```python
from build123d import *

# Parameters (mm, degrees)
F0_W     = 50.8
F0_H     = 38.1
F1_DEPTH = 50.8
F2_R     = 4.7625
F3_DEPTH = 50.801
F4_R     = 4.7625
F5_DEPTH = 38.101
F6_R     = 2.54
F7_DEPTH = 12.7
F8_R     = 2.54
F9_DEPTH = 19.05


with BuildPart() as f1:
    # F0 (on Front) → F1 (new body)
    with BuildSketch(Plane.XZ):
        Rectangle(F0_W, F0_H)
    extrude(amount=F1_DEPTH)

    # F2 (on face) → F3 (cut, through all)
    with BuildSketch(Plane(origin=(0, 0, 0), x_dir=(-1, 0, 0), z_dir=(0, 1, 0))):
        with Locations((-4.7625, 0)):
            Circle(F2_R)
    extrude(amount=-F3_DEPTH, mode=Mode.SUBTRACT)

    # F4 (on face) → F5 (cut, through all)
    with BuildSketch(Plane.XY.offset(19.05)):
        with Locations((-12.7, -25.4)):
            Circle(F4_R)
    extrude(amount=-F5_DEPTH, mode=Mode.SUBTRACT)

    # F6 (on face) → F7 (cut)
    with BuildSketch(Plane(origin=(-25.4, 0, 0), x_dir=(0, -1, 0), z_dir=(-1, 0, 0))):
        with Locations((25.4, 12.7)):
            Circle(F6_R)
    extrude(amount=-F7_DEPTH, mode=Mode.SUBTRACT)

    # F8 (on face) → F9 (cut)
    with BuildSketch(Plane.YZ.offset(25.4)):
        with Locations((-44.45, 0)):
            Circle(F8_R)
    extrude(amount=-F9_DEPTH, mode=Mode.SUBTRACT)


solid = f1.part
```
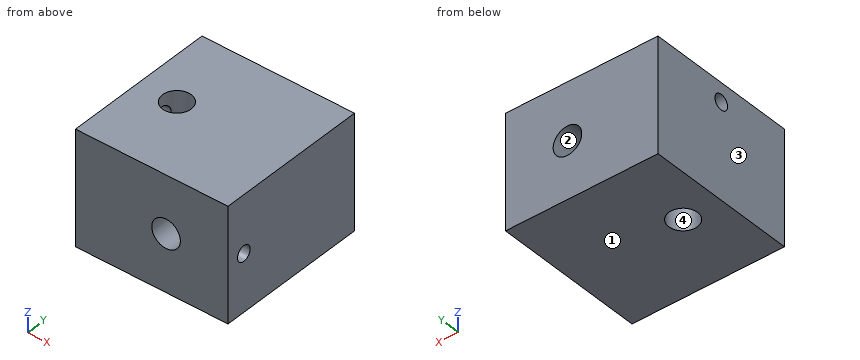
Check sheet for the modelled part. Datum: model origin and axes. Units: mm. Face numbers are marked on the shaded views. Give positions to 0.01 mm unless a question says otherwise; leave off trailing zeros. Write each loop counter-clockwise with the first axis right and the second up, starting at its lowest first coordinate (ties: lowest second). Pieces come first, ordered by that corner, then holes.
Item 1: Scan lines: L1, parallel to Z at x = -20.25, y = -25.4; L2, parallel to Y at x = 15, z = 0; L3, parallel to X at y = -28, z = 0 (3 decimals). Record each from-to range of solid material in increasing order.
Item 2: Cross-section at D-D (z = -13). Enter the section's corners in (x, y) (1 decimal), and give its area (3 significant figures).
Item 3: Cross-section at B-B (z = 0). Enter the section's corners in (x, y) (1 decimal), and give its area (3 significant figures).
Item 4: Cross-section at C-C (x = -14.5). Enter the section's corners in (y, z).
Item 5: Cross-section at A-A (y = -25.4). Count the separate pieces of the cut face and the enclosed holes in it, and give its area (3 significant figures).
Item 6: Draft check along X on the marked faces 1, 2, 3 and 4. Enter one of: released by +X, released by -X, zero draft, split by the parting line, or undercut.
Item 7: Gauge pin test, flat ends, axial feed: pin 1 (8 mm diameter, centred on x = 10, z = -12.5, fed in from +Y); pin 2 (7.5 mm diameter, centred on x = 4.76, z = 0, fed in from +Y) (1 decimal). Record the tip position at first contact, or that the pin passes through.
Report:
1. L1: z = -19.05 to 10.16, 15.24 to 19.05
1. L2: y = -50.8 to -46.99, -41.91 to 0
1. L3: x = -25.4 to -16.69, -8.71 to 0, 9.525 to 25.4
2. outline: (-25.4, -50.8) - (25.4, -50.8) - (25.4, 0) - (-25.4, 0) - close; hole circle Ø9.5 at (-12.7, -25.4)
2. area: 2,510 mm2
3. outline: (-25.4, -50.8) - (0, -50.8) - (0, 0) - (-25.4, 0) - close; (9.5, -50.8) - (25.4, -50.8) - (25.4, -47) - (9.5, -47) - close; (9.5, -41.9) - (25.4, -41.9) - (25.4, 0) - (9.5, 0) - close; hole circle Ø9.5 at (-12.7, -25.4)
3. area: 1,940 mm2
4. outline: (-50.8, -19.05) - (-29.81, -19.05) - (-29.81, 19.05) - (-50.8, 19.05) - close; (-20.99, -19.05) - (0, -19.05) - (0, 19.05) - (-20.99, 19.05) - close
5. separate pieces: 3
5. enclosed holes: 1
5. area: 1,460 mm2
6. face 1: zero draft
6. face 2: undercut
6. face 3: released by -X
6. face 4: undercut
7. pin 1: stops at y = 0
7. pin 2: passes through
